Read the model definition and answer for the solid it produces. Units are mm, in the model's axes. A direction names the side the tool comes from. Give positions to 0.01 mm unless a question says otherwise; leave off trailing zeros. Loops run counter-clockwise (first coordinate to the right, second up) from the corner with the lowest first, then second, coordinate; pieces in that order, holes last. Notation, with made-up numbers: (-32, -3) -> (22, -3) arc R30 cw to (22, 22) -> close; hole circle Ø2 at (-39.75, -0.5). An arc over 180 degrees is marked (long way). Write each question's results on one line, items separated by ' | '. Start each with the question number.
Item 1: Section B-B on y = -8 is taken. Write down the section's boundary in (x, z), and give its area (3 significant figures).
Item 2: Section C-C on x = -25 is taken. Write down the section's boundary in (y, z) (3 decimals), and give its area (3 significant figures).
Item 3: Each of these flat-tipped pins is pushed along its axis until it touches: P1, Ø1, axis at y = -132, z = 27, coming from the -X side; P2, Ø2.5, axis at x = 39.5, y = -148, coming from the +Z side; P3, Ø1, axis at x = 2, z = 8.5, coming from the -Y side (3 decimals). Where does it stop, or does it pass through?
Item 4: Which of the six approach directions +Z, -Z, +X, -X, +Y, -Y give full straight-line access (tool end or side, diameter ignored) to faces 1 (the flat face through (45, -116, 15)), 2 (the flat face through (0, -78, 1)), 3 (the flat face through (1, -53, 3)), 4 (the cylindrical face through (24.404, -136.185, 1.479)), 5 (the cylindrical face through (2.3, -152.3, 7.6))?
Item 5: Section D-D on y = -133.5 is taken. Write down the section's boundary in (x, z).
Item 6: Determine the mould class of faces 6 (the flat face through (-56.5, 5, 15)), 7 (the flat face through (-1, -31, 0)), 8 (the cylindrical face through (-25.759, -136.917, 1.479)), 9 (the flat face through (56.5, 4, 15)) for opening direction X: +X half, -X half, draft (parallel to the pull), parting line (faces both ways), or undercut.
Item 7: Section A-A on x = 17.5 is taken. Write down the section's boundary in (y, z) (3 decimals).
Item 8: Find the intervals of material crossed by line 1 (X direction, y = -117, z = 15.5); line 2 (Y direction, x = 19.5, z = 19.75) (3 decimals); line 3 (Y direction, x = -38, z = 1.75) (3 decimals), in increasing order.
```python
from build123d import *

# Parameters (mm, degrees)
SKETCH1_R           = 3.5
SKETCH1_R_2         = 2.75
SKETCH1_W           = 22
SKETCH1_H           = 5
SKETCH1_R_3         = 1.5
BOSS_EXTRUDE1_DEPTH = 30
CUT_EXTRUDE2_DEPTH  = 27
CUT_EXTRUDE4_DEPTH  = 1
FILLET1_R           = 2
BOSS_EXTRUDE2_DEPTH = 27
SKETCH6_R           = 1.5
CUT_EXTRUDE5_DEPTH  = 20
CUT_EXTRUDE6_REACH  = 210.53
SKETCH7_R           = 7.75


with BuildPart() as part:
    # Sketch1 → Boss-Extrude1 (new body)
    with BuildSketch(Plane.XY):
        Polygon((56.5, 44.975), (-56.5, 44.975), (-56.5, -34.975), (-45, -78.5), (-45, -153.5), (45, -153.5), (45, -78.5), (56.5, -34.975), align=None)
        with Locations((-25, -133.5)):
            Circle(SKETCH1_R, mode=Mode.SUBTRACT)
        with Locations((-40, -58.5)):
            Circle(SKETCH1_R_2, mode=Mode.SUBTRACT)
        with Locations((0, -121)):
            Rectangle(SKETCH1_W, SKETCH1_H, mode=Mode.SUBTRACT)
        with Locations((25, -133.5)):
            Circle(SKETCH1_R_2, mode=Mode.SUBTRACT)
        with Locations((40, -58.5)):
            Circle(SKETCH1_R_2, mode=Mode.SUBTRACT)
        with Locations((-43.9, -32.375)):
            Circle(SKETCH1_R_3, mode=Mode.SUBTRACT)
        with Locations((-43.9, 32.375)):
            Circle(SKETCH1_R_3, mode=Mode.SUBTRACT)
        with Locations((43.9, -32.375)):
            Circle(SKETCH1_R_3, mode=Mode.SUBTRACT)
        Polygon((-39.25, -25.5), (-39.25, 25.5), (39.25, 25.5), (39.25, 21.45), (43.95, 21.45), (43.95, -21.45), (39.25, -21.45), (39.25, -25.5), align=None, mode=Mode.SUBTRACT)
        with Locations((43.9, 32.375)):
            Circle(SKETCH1_R_3, mode=Mode.SUBTRACT)
    extrude(amount=BOSS_EXTRUDE1_DEPTH)

    # Sketch2 → Cut-Extrude2 (cut)
    with BuildSketch(Plane.XY.offset(30)):
        Polygon((54, 42.475), (54, -34.65030126), (42.5, -78.17530126), (42.5, -151), (-42.5, -151), (-42.5, -78.17530126), (-54, -34.65030126), (-54, 42.475), align=None)
    extrude(amount=-CUT_EXTRUDE2_DEPTH, mode=Mode.SUBTRACT)

    # Sketch1<3> → Cut-Extrude4 (cut)
    with BuildSketch(Plane.XY):
        with BuildLine():
            Line((-28, -118.5), (28, -118.5))
            ThreePointArc((28, -118.5), (32.949747468, -116.449747468), (35, -111.5))
            Line((35, -111.5), (35, -45.5))
            ThreePointArc((35, -45.5), (32.949747468, -40.550252532), (28, -38.5))
            Line((28, -38.5), (-28, -38.5))
            ThreePointArc((-28, -38.5), (-32.949747468, -40.550252532), (-35, -45.5))
            Line((-35, -45.5), (-35, -111.5))
            ThreePointArc((-35, -111.5), (-32.949747468, -116.449747468), (-28, -118.5))
        make_face()
    extrude(amount=CUT_EXTRUDE4_DEPTH, mode=Mode.SUBTRACT)

    # Fillet1
    fillet1_edges = [part.edges().sort_by_distance(p)[0] for p in [
        (56.5, 44.975, 15),
        (56.5, -34.975, 15),
        (45, -78.5, 15),
        (45, -153.5, 15),
        (-45, -153.5, 15),
        (-45, -78.5, 15),
        (-56.5, -34.975, 15),
        (-56.5, 44.975, 15),
    ]]
    fillet(fillet1_edges, radius=FILLET1_R)

    # Sketch5 → Boss-Extrude2 (add, through all)
    with BuildSketch(Plane.XY.offset(3)):
        with BuildLine():
            Line((-42.5, -151), (-42.5, -148))
            ThreePointArc((-42.5, -148), (-37.378679656, -145.878679656), (-39.5, -151))
            Line((-39.5, -151), (-42.5, -151))
        make_face()
        with BuildLine():
            Line((39.5, -151), (42.5, -151))
            Line((42.5, -151), (42.5, -148))
            ThreePointArc((42.5, -148), (37.378679656, -145.878679656), (39.5, -151))
        make_face()
        with BuildLine():
            Line((-54, 42.475), (-51, 42.475))
            ThreePointArc((-51, 42.475), (-48.878679656, 37.353679656), (-54, 39.475))
            Line((-54, 39.475), (-54, 42.475))
        make_face()
        with BuildLine():
            Line((54, 39.475), (54, 42.475))
            Line((54, 42.475), (51, 42.475))
            ThreePointArc((51, 42.475), (48.878679656, 37.353679656), (54, 39.475))
        make_face()
    extrude(amount=BOSS_EXTRUDE2_DEPTH)

    # Sketch6 → Cut-Extrude5 (cut)
    with BuildSketch(Plane.XY.offset(30)):
        with Locations((51, 39.475)):
            Circle(SKETCH6_R)
        with Locations((39.5, -148)):
            Circle(SKETCH6_R)
        with Locations(Location((-39.5, -148, 0), (0, 0, 180))):
            Circle(SKETCH6_R)
        with Locations(Location((-51, 39.475, 0), (0, 0, 180))):
            Circle(SKETCH6_R)
    extrude(amount=-CUT_EXTRUDE5_DEPTH, mode=Mode.SUBTRACT)

    # Sketch7 → Cut-Extrude6 (cut, up to next)
    with BuildSketch(Plane.XZ.offset(153.5), mode=Mode.PRIVATE) as cut_extrude6_sk1:
        with Locations(Location((0, 15, 0), (0, 0, 270))):
            Circle(SKETCH7_R)
    cut_extrude6_tool1 = extrude(cut_extrude6_sk1.sketch, amount=-CUT_EXTRUDE6_REACH, mode=Mode.PRIVATE) & part.part
    add(cut_extrude6_tool1.solids().sort_by_distance((0, -153.5, 15))[0], mode=Mode.SUBTRACT)


solid = part.part
```
Findings:
1) outline: (-56.5, 0) -> (-39.25, 0) -> (-39.25, 3) -> (-54, 3) -> (-54, 30) -> (-56.5, 30) -> close; (43.95, 0) -> (56.5, 0) -> (56.5, 30) -> (54, 30) -> (54, 3) -> (43.95, 3) -> close | area: 224 mm2
2) outline: (-153.5, 0) -> (-137, 0) -> (-137, 3) -> (-151, 3) -> (-151, 30) -> (-153.5, 30) -> close; (-130, 0) -> (-118.5, 0) -> (-118.5, 1) -> (-38.5, 1) -> (-38.5, 0) -> (-25.5, 0) -> (-25.5, 3) -> (-130, 3) -> close; (25.5, 0) -> (44.975, 0) -> (44.975, 30) -> (42.475, 30) -> (42.475, 3) -> (25.5, 3) -> close | area: 476 mm2
3) P1: x = -45 | P2: z = 10 | P3: y = 42.475
4) face 1: +Z, -Z, +X, -Y | face 2: -Z | face 3: +Z | face 4: +Z, -Z | face 5: -Y
5) outline: (-45, 0) -> (-28.5, 0) -> (-28.5, 3) -> (-42.5, 3) -> (-42.5, 30) -> (-45, 30) -> close; (-21.5, 0) -> (22.25, 0) -> (22.25, 3) -> (-21.5, 3) -> close; (27.75, 0) -> (45, 0) -> (45, 30) -> (42.5, 30) -> (42.5, 3) -> (27.75, 3) -> close
6) face 6: -X half | face 7: draft | face 8: undercut | face 9: +X half
7) outline: (-153.5, 0) -> (-118.5, 0) -> (-118.5, 1) -> (-38.5, 1) -> (-38.5, 0) -> (-25.5, 0) -> (-25.5, 3) -> (-151, 3) -> (-151, 30) -> (-153.5, 30) -> close; (25.5, 0) -> (44.975, 0) -> (44.975, 30) -> (42.475, 30) -> (42.475, 3) -> (25.5, 3) -> close
8) line 1: -45 to -42.5, 42.5 to 45 | line 2: -153.5 to -151, 42.475 to 44.975 | line 3: -153.5 to -60.387, -56.613 to -25.5, 25.5 to 44.975
